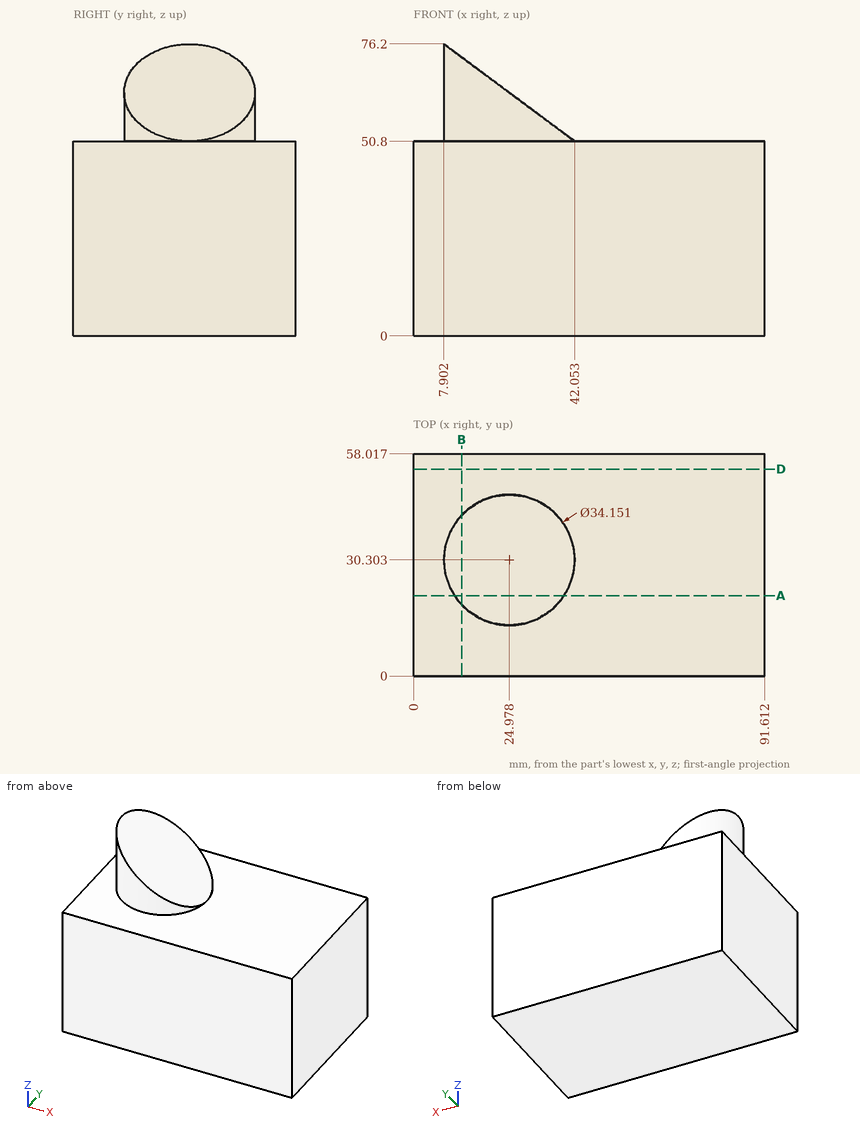
Design review of the part shown in the three views and the two pictorial views. Dimensions are in mm from the part's minimum x, y and z. Round coordinates to 2 decimals unless told otherwise and drop trailing zeros. Loops run counter-clockwise (first coordinate to the right, second up) from the corner with the lowest first, then second, coordinate; pieces in that order, holes last.
Q1. To check wall thickness, follow line 1 along Z through (x, y) = (66.5, 33); line 2 along Z through (x, y) = (13.5, 26.5) (1 decimal); line 3 along Y through (x, z) = (28, 51). State the ranges of each line that lie inside material, in increasing order.
Result sheet:
line 1: z = 0 to 50.8
line 2: z = 0 to 72
line 3: y = 13.5 to 47.11
Q2. Insertion check: pin 1 Ø12 at (x, y) = (58.5, 28.5) entering from +Z; pin 2 Ø5 at (y, z) = (12.5, 62) entering from -X; pin 3 Ø4 at (y, z) = (32.5, 60.5) entering from -X. Each pin has a flat end and moves straight along its axis. Give the tip position at first contact, or say it passes through.
Result sheet:
pin 1: stops at z = 50.8
pin 2: stops at x = 17.4
pin 3: stops at x = 7.9
Q3. Add section D-D on y = 54. Write out the cut boundary in (x, z), plus the area to 3 significant figures.
Result sheet:
outline: (0, 0) - (91.61, 0) - (91.61, 50.8) - (0, 50.8) - close
area: 4,650 mm2
Q4. Add section A-A on y = 21. Write out the cut boundary in (x, z).
Result sheet:
outline: (0, 0) - (91.61, 0) - (91.61, 50.8) - (39.3, 50.8) - (39.3, 52.85) - (10.66, 74.15) - (10.66, 50.8) - (0, 50.8) - close
Q5. Add section B-B on x = 12.5. Write out the cut boundary in (y, z), plus the area to 3 significant figures.
Result sheet:
outline: (0, 0) - (58.02, 0) - (58.02, 50.8) - (41.96, 50.8) - (41.96, 72.78) - (18.65, 72.78) - (18.65, 50.8) - (0, 50.8) - close
area: 3,460 mm2
